Source: CAD feature listing. Evaluate the final solid. Frame: model axes, mm. A direction names the side the tool comes from. Give positions to 0.01 mm unless a question says otherwise; leave off trailing zeros. Order: outer loops, then holes, each group sorted by start corner. A loop starts at its lowest first (then second) coordinate and runs counter-clockwise, first axis right, second up. Notation, with made-up numbers: M 50.25,87 L 54.25,87 A16 cw 54.25,100 Z; hole C 46,43.5 d4. An arc over 180 degrees is marked long. Answer in a Markdown table with one row per item. Add a question column.
(1) Section query D-D, the plane z = 6.5. Return loops of the section in (x, y).
(2) Material intervals for line 1 along Y through (x, z) = (29, 4); line 2 along Y through (x, z) = (-29, 1.6); line 3 along Y through (x, z) = (5, 1), sorted ascending.
(3) Set-up query: faces 4 (the face through (25.789, 25.696, 6.479)), 5 (the face through (-14.859, 14.797, 4.056)), 6 (the face through (27.6, 27.6, 3.4)). Return all of +Z, -Z, +X, -X, +Y, -Y with unobstructed straight access to the full face (end or side cutting, diameter ignored); none if empty.
(4) Mould query, pull axis X, two halves, no side actions, for faces 1 (the face through (0, -39, 2)), 2 (the face through (32, 0, 2)), 3 (the face through (-30.5, 26.117, 1.676)). Classes: pulls with the +X half, pulls with the -X half, needs draft (parallel to the pull), parting line crosses it, or undercut.
(5) Pin query (flat end, axial travel): P1, Ø3, axis at x = -29.5, y = 30, coming from the -Z side; P2, Ø5, axis at x = 29, y = -29, coming from the +Z side; P3, Ø10, axis at x = -8.5, y = 26, coming from the -Z side; P4, Ø3.5, axis at y = 10, z = 7, coming from the +X side. Return the tip coordinate at first contact, or that it passes through.
(6) Section query B-B, the plane z = 2. Count the separate pieces of the cut face and the enclosed holes in it, plus the area to 3 significant figures.
(7) Section query C-C, the plane x = -7. Return loops of the section in (y, z).
(8) Section query A-A, the plane y = 2.5. Return loops of the section in (x, z).
from build123d import *

# Parameters (mm, degrees)
BOSS_EXTRUDE1_DEPTH                                 = 5
BOSS_EXTRUDE2_DEPTH                                 = 3
CUT_EXTRUDE1_DEPTH                                  = 56.731499172
CUT_EXTRUDE1_DEPTH_BACK                             = 56.731499172
CBORE_FOR_M3_HEX_SOCKET_HEAD_CAP_SCREW1_D           = 3.2
CBORE_FOR_M3_HEX_SOCKET_HEAD_CAP_SCREW1_CBORE_D     = 6.5
CBORE_FOR_M3_HEX_SOCKET_HEAD_CAP_SCREW1_CBORE_DEPTH = 3.4


with BuildPart() as part:
    # Sketch1 → Boss-Extrude1 (new body)
    with BuildSketch(Plane.XY):
        with BuildLine():
            Line((-29, 39), (29, 39))
            ThreePointArc((29, 39), (36.071067812, 36.071067812), (39, 29))
            Line((39, 29), (39, 17.5))
            Line((39, 17.5), (34.928932188, 13.428932188))
            ThreePointArc((34.928932188, 13.428932188), (32.761204675, 10.1846987), (32, 6.357864376))
            Line((32, 6.357864376), (32, -6.357864376))
            ThreePointArc((32, -6.357864376), (32.761204675, -10.1846987), (34.928932188, -13.428932188))
            Line((34.928932188, -13.428932188), (39, -17.5))
            Line((39, -17.5), (39, -29))
            ThreePointArc((39, -29), (36.071067812, -36.071067812), (29, -39))
            Line((29, -39), (-29, -39))
            ThreePointArc((-29, -39), (-36.071067812, -36.071067812), (-39, -29))
            Line((-39, -29), (-39, -17.5))
            Line((-39, -17.5), (-34.928932188, -13.428932188))
            ThreePointArc((-34.928932188, -13.428932188), (-32.761204675, -10.1846987), (-32, -6.357864376))
            Line((-32, -6.357864376), (-32, 6.357864376))
            ThreePointArc((-32, 6.357864376), (-32.761204675, 10.1846987), (-34.928932188, 13.428932188))
            Line((-34.928932188, 13.428932188), (-39, 17.5))
            Line((-39, 17.5), (-39, 29))
            ThreePointArc((-39, 29), (-36.071067812, 36.071067812), (-29, 39))
        make_face()
    extrude(amount=BOSS_EXTRUDE1_DEPTH)

    # Sketch2 → Boss-Extrude2 (add)
    with BuildSketch(Plane(origin=(0, 0, 5), x_dir=(-1, 0, 0), z_dir=(0, 0, -1))):
        with BuildLine():
            Line((-21.5, 27.5), (21.5, 27.5))
            ThreePointArc((21.5, 27.5), (25.742640687, 25.742640687), (27.5, 21.5))
            Line((27.5, 21.5), (27.5, -21.5))
            ThreePointArc((27.5, -21.5), (25.742640687, -25.742640687), (21.5, -27.5))
            Line((21.5, -27.5), (-21.5, -27.5))
            ThreePointArc((-21.5, -27.5), (-25.742640687, -25.742640687), (-27.5, -21.5))
            Line((-27.5, -21.5), (-27.5, 21.5))
            ThreePointArc((-27.5, 21.5), (-25.742640687, 25.742640687), (-21.5, 27.5))
        make_face()
    extrude(amount=-BOSS_EXTRUDE2_DEPTH)

    # Sketch3 → Cut-Extrude1 (cut, two sides: drawn at the far end of the back side and taken through both)
    with BuildSketch(Plane(origin=(0, 0, 0), x_dir=(-1, 0, 0), z_dir=(0, 0, -1)).offset(-CUT_EXTRUDE1_DEPTH_BACK)):
        with BuildLine():
            Line((-12, -16), (12, -16))
            ThreePointArc((12, -16), (14.828427125, -14.828427125), (16, -12))
            Line((16, -12), (16, 12))
            ThreePointArc((16, 12), (14.828427125, 14.828427125), (12, 16))
            Line((12, 16), (-12, 16))
            ThreePointArc((-12, 16), (-14.828427125, 14.828427125), (-16, 12))
            Line((-16, 12), (-16, -12))
            ThreePointArc((-16, -12), (-14.828427125, -14.828427125), (-12, -16))
        make_face()
    extrude(amount=CUT_EXTRUDE1_DEPTH + CUT_EXTRUDE1_DEPTH_BACK, mode=Mode.SUBTRACT)

    # CBORE for M3 Hex Socket Head Cap Screw1 (through all)
    with Locations(Plane(origin=(0, 0, 0), x_dir=(-1, 0, 0), z_dir=(0, 0, -1))):
        with Locations((29, -29), (29, 29), (-29, 29), (-29, -29)):
            CounterBoreHole(CBORE_FOR_M3_HEX_SOCKET_HEAD_CAP_SCREW1_D / 2, CBORE_FOR_M3_HEX_SOCKET_HEAD_CAP_SCREW1_CBORE_D / 2, CBORE_FOR_M3_HEX_SOCKET_HEAD_CAP_SCREW1_CBORE_DEPTH)


solid = part.part
Values follow:
| question | item | result |
|---|---|---|
| 1 | outline | M -27.5,-21.5 A6 ccw -21.5,-27.5 L 21.5,-27.5 A6 ccw 27.5,-21.5 L 27.5,21.5 A6 ccw 21.5,27.5 L -21.5,27.5 A6 ccw -27.5,21.5 Z; hole M -16,-12 A4 ccw -12,-16 L 12,-16 A4 ccw 16,-12 L 16,12 A4 ccw 12,16 L -12,16 A4 ccw -16,12 Z |
| 2 | line 1 | y = -39 to -30.6, -27.4 to 27.4, 30.6 to 39 |
| 2 | line 2 | y = -39 to -32.25, -25.75 to 25.75, 32.25 to 39 |
| 2 | line 3 | y = -39 to -16, 16 to 39 |
| 3 | face 4 | +Z, +X, +Y |
| 3 | face 5 | +Z, -Z |
| 3 | face 6 | -Z |
| 4 | face 1 | needs draft |
| 4 | face 2 | pulls with the +X half |
| 4 | face 3 | undercut |
| 5 | P1 | stops at z = 3.4 |
| 5 | P2 | stops at z = 5 |
| 5 | P3 | stops at z = 0 |
| 5 | P4 | stops at x = 27.5 |
| 6 | separate pieces | 1 |
| 6 | enclosed holes | 5 |
| 6 | area | 4,470 mm² |
| 7 | outline | M -39,0 L -16,0 L -16,8 L -27.5,8 L -27.5,5 L -39,5 Z; M 16,0 L 39,0 L 39,5 L 27.5,5 L 27.5,8 L 16,8 Z |
| 8 | outline | M -32,0 L -16,0 L -16,8 L -27.5,8 L -27.5,5 L -32,5 Z; M 16,0 L 32,0 L 32,5 L 27.5,5 L 27.5,8 L 16,8 Z |
